Here's how the part is built. I have some questions about the finished solid (model axes, mm). A direction names the side the tool comes from. Round coordinates to 2 decimals unless told otherwise and drop trailing zeros. Order: outer loops, then holes, each group sorted by start corner. A loop starts at its lowest first (then second) coordinate and runs counter-clockwise, first axis right, second up.
```python
from build123d import *

# Parameters (mm, degrees)
EXTRUDE_1_DEPTH     = 7
SKETCH_2_R          = 1.499068593
SKETCH_2_R_2        = 1.507712359
CUT_EXTRUDE_1_DEPTH = 2
SKETCH_3_R          = 1.404162934
SKETCH_3_R_2        = 1.394662516
SKETCH_3_R_3        = 1.426202715
SKETCH_3_R_4        = 1.43
CUT_EXTRUDE_2_DEPTH = 2
SKETCH_5_W          = 8
SKETCH_5_H          = 5
CUT_EXTRUDE_3_DEPTH = 135
SKETCH_6_W          = 48
SKETCH_6_H          = 2
SKETCH_6_W_2        = 38.5
EXTRUDE_2_DEPTH     = 8.5
SKETCH_7_W          = 16
SKETCH_7_H          = 11.5
EXTRUDE_3_DEPTH     = 10
SKETCH_9_W          = 2
SKETCH_9_H          = 8.5
CUT_EXTRUDE_4_DEPTH = 10
SKETCH_10_W         = 9
SKETCH_10_H         = 11
EXTRUDE_4_DEPTH     = 3
EXTRUDE_5_DEPTH     = 10.5
SKETCH_12_R         = 1.404162934
SKETCH_12_R_2       = 1.394662516
SKETCH_12_R_3       = 1.451975752
SKETCH_12_R_4       = 1.426202713
CUT_EXTRUDE_5_DEPTH = 10.5


with BuildPart() as part:
    # Sketch 1 → Extrude 1 (new body)
    with BuildSketch(Plane(origin=(0, 0, 0), x_dir=(1, 0, 0), z_dir=(0, 1, 0))):
        Polygon((0, 15.813216669), (3.578877576, 19.392094245), (3.578877576, 50.54921212), (0, 52.598301515), (0, 57), (-78, 57), (-78, 0), (0, 0), align=None)
    extrude(amount=EXTRUDE_1_DEPTH)

    # Sketch 2 → Cut-Extrude 1 (cut)
    with BuildSketch(Plane(origin=(0, 7, 0), x_dir=(1, 0, 0), z_dir=(0, 1, 0))):
        with Locations((-73.839384245, 53.362286428)):
            Circle(SKETCH_2_R)
        with Locations((-73.839384245, 4.894512841)):
            Circle(SKETCH_2_R_2)
    extrude(amount=-CUT_EXTRUDE_1_DEPTH, mode=Mode.SUBTRACT)

    # Sketch 3 → Cut-Extrude 2 (cut)
    with BuildSketch(Plane(origin=(0, 7, 0), x_dir=(1, 0, 0), z_dir=(0, 1, 0))):
        with Locations((-55.116977268, 52.270174236)):
            Circle(SKETCH_3_R)
        with Locations((-55.116977268, 6.180833795)):
            Circle(SKETCH_3_R_2)
        with Locations((-2.023984121, 48.167273678)):
            Circle(SKETCH_3_R_3)
        with Locations((-2.023984121, 22.405667973)):
            Circle(SKETCH_3_R_4)
    extrude(amount=-CUT_EXTRUDE_2_DEPTH, mode=Mode.SUBTRACT)

    # Sketch 5 → Cut-Extrude 3 (cut)
    with BuildSketch(Plane.XY):
        with Locations((-74, 2.5)):
            Rectangle(SKETCH_5_W, SKETCH_5_H)
    extrude(amount=-CUT_EXTRUDE_3_DEPTH, mode=Mode.SUBTRACT)

    # Sketch 6 → Extrude 2 (add)
    with BuildSketch(Plane(origin=(0, 0, 0), x_dir=(-1, 0, 0), z_dir=(0, -1, 0))):
        with Locations((26.66066087, 3.286523813)):
            Rectangle(SKETCH_6_W, SKETCH_6_H)
        with Locations((21.91066087, 54.141974349)):
            Rectangle(SKETCH_6_W_2, SKETCH_6_H)
    extrude(amount=EXTRUDE_2_DEPTH)

    # Sketch 7 → Extrude 3 (add)
    with BuildSketch(Plane(origin=(0, 0, 0), x_dir=(-1, 0, 0), z_dir=(0, -1, 0))):
        with Locations((67.251369974, 18.045913209)):
            Rectangle(SKETCH_7_W, SKETCH_7_H)
    extrude(amount=EXTRUDE_3_DEPTH)

    # Sketch 9 → Cut-Extrude 4 (cut)
    with BuildSketch(Plane.ZY.offset(41.16066087)):
        with Locations((-54.141974349, -4.25)):
            Rectangle(SKETCH_9_W, SKETCH_9_H)
    extrude(amount=-CUT_EXTRUDE_4_DEPTH, mode=Mode.SUBTRACT)



with BuildPart() as body_2:
    # Sketch 10 → Extrude 4 (new body)
    with BuildSketch(Plane.ZY.offset(70)):
        with Locations((-49.837173762, -5.5)):
            Rectangle(SKETCH_10_W, SKETCH_10_H)
    extrude(amount=-EXTRUDE_4_DEPTH)


with BuildPart() as part_1:
    add(part.part)

    add(body_2.part)  # Extrude 5 merges body 2
    # Sketch 11 → Extrude 5 (add)
    with BuildSketch(Plane(origin=(-67, 0, 0), x_dir=(0, 0, -1), z_dir=(1, 0, 0))):
        with BuildLine():
            Line((45.337173762, 0), (54.337173762, 0))
            Line((54.337173762, 0), (54.337173762, -6.5))
            ThreePointArc((54.337173762, -6.5), (49.837173762, -11), (45.337173762, -6.5))
            Line((45.337173762, -6.5), (45.337173762, 0))
        make_face()
    extrude(amount=EXTRUDE_5_DEPTH)

    # Sketch 12 → Cut-Extrude 5 (cut)
    with BuildSketch(Plane(origin=(0, 5, 0), x_dir=(1, 0, 0), z_dir=(0, 1, 0))):
        with Locations((-55.116977268, 52.270174236)):
            Circle(SKETCH_12_R)
        with Locations((-55.116977268, 6.180833795)):
            Circle(SKETCH_12_R_2)
        with Locations((-2.040608488, 22.420040311)):
            Circle(SKETCH_12_R_3)
        with Locations((-2.023984121, 48.167273678)):
            Circle(SKETCH_12_R_4)
    extrude(amount=-CUT_EXTRUDE_5_DEPTH, mode=Mode.SUBTRACT)


solid = part_1.part
```
1. I need wall thicknesses on probe 1 along X at (y, z) = (-5, -53.5); probe 2 along Z at (x, y) = (-69, -4.5); probe 3 along Y at (x, z) = (-30, -50). Which ranges of each line are inside material? Lowest first, please.
Evaluation:
probe 1: x = -70 to -56.5, -31.16 to -2.66
probe 2: z = -54.34 to -45.34, -23.8 to -12.3
probe 3: y = 0 to 7
2. If we section it at B-B, the plane x = -43: Write out the boundary of the cut face in (y, z).
Evaluation:
outline: (-8.5, -4.29) - (0, -4.29) - (0, -57) - (7, -57) - (7, 0) - (0, 0) - (0, -2.29) - (-8.5, -2.29) - close
3. I'm going to push flat-ended pins straight in: P1, Ø1.7, axis at x = -55.12, z = -52.27, coming from the -Y side; P2, Ø6, axis at x = -20.5, z = -23, coming from the -Y side; P3, Ø5, axis at y = -7, z = -6.5, coming from the +X side; P4, Ø5.5, axis at x = -60.5, y = -3.5, coming from the -Z side. Where does each tip first touch, or does it pass through?
Evaluation:
P1: passes through
P2: stops at y = 0
P3: stops at x = -2.66
P4: stops at z = -54.34
4. If we section it at D-D, the plane z = -17: Write out the boundary of the cut face in (x, y), and give its area (3 significant figures).
Evaluation:
outline: (-78, 5) - (-70, 5) - (-70, 0) - (-75.25, 0) - (-75.25, -10) - (-59.25, -10) - (-59.25, 0) - (1.19, 0) - (1.19, 7) - (-78, 7) - close
area: 674 mm2
5. If we section it at C-C, the plane z = -31.5: Write out the boundary of the cut face in (x, y), and give its area (3 significant figures).
Evaluation:
outline: (-78, 5) - (-70, 5) - (-70, 0) - (3.58, 0) - (3.58, 7) - (-78, 7) - close
area: 531 mm2
6. On a 3-axis mill with a long thin cutter (end or side, diameter ignored), from which of +Z, -Z, +X, -X, +Y, -Y can I reach the whole of each face in a straight line? I mean faces 5 (the flat face through (-17, -8.5, -54)), 6 (the flat face through (-17, -4, -55.142)), 7 (the flat face through (-65, -4, -45.337)), 8 (the flat face through (0, 3, -55)), 9 (the flat face through (-26, -4, -2.287)). Say none if no direction works.
Evaluation:
face 5: +Z, -Z, +X, -Y
face 6: -Z, +X, -X, -Y
face 7: +X, -X, -Y
face 8: -Z, +X, +Y, -Y
face 9: +Z, +X, -X, -Y
7. If we section it at A-A, the plane y = -3.5: Write out the boundary of the cut face in (x, z).
Evaluation:
outline: (-75.25, -23.8) - (-59.25, -23.8) - (-59.25, -12.3) - (-75.25, -12.3) - close; (-70, -54.34) - (-56.5, -54.34) - (-56.5, -52.51) arc R1.4 cw to (-56.5, -52.03) - (-56.5, -45.34) - (-70, -45.34) - close; (-50.66, -4.29) - (-2.66, -4.29) - (-2.66, -2.29) - (-50.66, -2.29) - close; (-31.16, -55.14) - (-2.66, -55.14) - (-2.66, -53.14) - (-31.16, -53.14) - close
8. If we mould it in two halves opening along Y, with no side actions, what happens to faces 1 (the flat face through (-70, 0.4, -34.4)), 2 (the cylindrical face through (-2.23, 2.54, -23.86)), 3 (the flat face through (-67, -10, -18)), 4 (the flat face through (-74, 5, -28))? For each: released by +Y, released by -Y, zero draft, split by the parting line, or undercut.
Evaluation:
face 1: undercut
face 2: zero draft
face 3: released by -Y
face 4: undercut
